```python
from build123d import *

# Parameters (mm, degrees)
ODEBRAT_VYSUNUT_M1_DEPTH = 2.4
ODEBRAT_VYSUNUT_M2_DEPTH = 2.9
SKICA4_W                 = 43.201709197
SKICA4_H                 = 57.022390215
SKICA4_W_2               = 28.704491345
SKICA4_H_2               = 62.531332999
ODEBRAT_VYSUNUT_M3_DEPTH = 320.0000001
M6_Z_VIT1_D              = 5
M6_Z_VIT1_DEPTH          = 22
M6_Z_VIT1_TIP            = 1.502151548
M5_Z_VIT1_D              = 4.2
M5_Z_VIT1_DEPTH          = 20
M5_Z_VIT1_TIP            = 1.2618073
ZKOSEN_1_SIZE            = 1
ZKOSEN_1_SIZE2           = 0.577350269
ZKOSEN_1_PART_2_SIZE     = 1
ZKOSEN_1_PART_2_SIZE2    = 0.577350269


with BuildPart() as part:
    # Skica1 → Rotovat1 (revolve)
    with BuildSketch(Plane.XY, mode=Mode.PRIVATE) as rotovat1_sk:
        Polygon((0, 0), (0, 6), (39, 6), (39, 5.75), (83.5, 5.75), (83.5, 6), (113.5, 6), (113.5, 5.75), (158, 5.75), (158, 6), (174, 6), (174, 10), (184, 10), (184, 9.75), (286.5, 9.75), (286.5, 10), (310, 10), (310, 12.5), (319, 12.5), (319, 10), (329, 10), (329, 9.75), (570, 9.75), (570, 7.5), (630, 7.5), (630, 6), (642, 6), (642, 0), align=None)
    revolve(rotovat1_sk.sketch.rotate(Axis((-5427.299905209, 0, 0), (1, 0, 0)), 180), axis=Axis((-5427.299905209, 0, 0), (1, 0, 0)))  # turned: the seam where the file's is

    # Skica2 → Odebrat vysunutím1 (cut)
    with BuildSketch(Plane(origin=(0, 6, 0), x_dir=(1, 0, 0), z_dir=(0, 1, 0))):
        with BuildLine():
            Line((6, 2), (18, 2))
            ThreePointArc((18, 2), (20, 0), (18, -2))
            Line((18, -2), (6, -2))
            ThreePointArc((6, -2), (4, 0), (6, 2))
        make_face()
    extrude(amount=-ODEBRAT_VYSUNUT_M1_DEPTH, mode=Mode.SUBTRACT)

    # Skica3 → Odebrat vysunutím2 (cut)
    with BuildSketch(Plane(origin=(0, 7.5, 0), x_dir=(1, 0, 0), z_dir=(0, 1, 0))):
        with BuildLine():
            Line((616, 2.5), (623, 2.5))
            ThreePointArc((623, 2.5), (625.5, 0), (623, -2.5))
            Line((623, -2.5), (616, -2.5))
            ThreePointArc((616, -2.5), (613.5, 0), (616, 2.5))
        make_face()
    extrude(amount=-ODEBRAT_VYSUNUT_M2_DEPTH, mode=Mode.SUBTRACT)

    # Skica4 → Odebrat vysunutím3 (cut, through all)
    with BuildSketch(Plane(origin=(319, 0, 0), x_dir=(0, 0, -1), z_dir=(1, 0, 0))):
        with Locations((-32.600854599, -5.674005363)):
            Rectangle(SKICA4_W, SKICA4_H)
        with Locations((25.352245673, -4.175959518)):
            Rectangle(SKICA4_W_2, SKICA4_H_2)
    extrude(amount=-ODEBRAT_VYSUNUT_M3_DEPTH, mode=Mode.SUBTRACT)

    # M6 závit1
    with Locations(Plane(origin=(642, 0, 0), x_dir=(0, 0, -1), z_dir=(1, 0, 0))):
        with Locations((0, 0)):
            Hole(M6_Z_VIT1_D / 2, depth=M6_Z_VIT1_DEPTH)
            with Locations((0, 0, -(M6_Z_VIT1_DEPTH + M6_Z_VIT1_TIP / 2))):  # 118° drill point
                Cone(0, M6_Z_VIT1_D / 2, M6_Z_VIT1_TIP, mode=Mode.SUBTRACT)

    # M5 závit1
    with Locations(Plane.ZY):
        with Locations((0, 0)):
            Hole(M5_Z_VIT1_D / 2, depth=M5_Z_VIT1_DEPTH)
            with Locations((0, 0, -(M5_Z_VIT1_DEPTH + M5_Z_VIT1_TIP / 2))):  # 118° drill point
                Cone(0, M5_Z_VIT1_D / 2, M5_Z_VIT1_TIP, mode=Mode.SUBTRACT)

    # Zkosení1
    zkosen_1_edges = [part.edges().sort_by_distance(p)[0] for p in [
        (570, 9.75, 0),
    ]]
    zkosen_1_side = [part.faces().sort_by_distance(p)[0] for p in [
        (449.5, 9.75, 0),
    ]]
    chamfer(zkosen_1_edges, length=ZKOSEN_1_SIZE, length2=ZKOSEN_1_SIZE2, reference=zkosen_1_side[0])

    # Zkosení1 part 2
    zkosen_1_part_2_edges = [part.edges().sort_by_distance(p)[0] for p in [
        (174, 10, 0),
    ]]
    zkosen_1_part_2_side = [part.faces().sort_by_distance(p)[0] for p in [
        (179, 10, 0),
    ]]
    chamfer(zkosen_1_part_2_edges, length=ZKOSEN_1_PART_2_SIZE, length2=ZKOSEN_1_PART_2_SIZE2, reference=zkosen_1_part_2_side[0])


solid = part.part
```
Model file for the job. Use its own axes, mm. A direction names the side the tool comes from. Coordinates: 2 decimals unless noted, no trailing zeros. Loops run counter-clockwise (first coordinate to the right, second up) from the corner with the lowest first, then second, coordinate; pieces in that order, holes last. Notation, with made-up numbers: (25, 31) - (75, 31) arc R33 cw to (75, 59) - close; hole circle Ø2 at (0, 13). An arc over 180 degrees is marked (long way). Write item = value, one per line. Start each with the question number.
Item 1: Saw through at A-A, the plane x = 337. List the corners of the cut face in (y, z), then the cut area to 3 significant figures.
Item 2: 3-axis set-ups, long thin cutter, end or side, ignore diameter. For faces 1 (the face through (298, 10, 0)), 2 (the face through (570, 8, 0)), 3 (the face through (0, 3, 0)): which of +Z, -Z, +X, -X, +Y, -Y reach the whole face in a straight line?
Item 3: Drop flat-ended pins along their axis: pin 1 Ø1 at (x, y) = (424, -1.5) entering from -Z; pin 2 Ø8 at (x, z) = (298.5, -4.5) entering from +Y; pin 3 Ø1.5 at (x, z) = (360, -3.5) entering from +Y. Give the stop position or say it passes through.
Item 4: Wall check: probe 1 along X at (y, z) = (1.25, 5.75); probe 2 along Z at (x, y) = (632.25, 0); probe 3 along Z at (x, y) = (11.75, 0). Give the ranges that are in metal, low to high. Write a range as [from, to].
Answers:
q1.outline = circle Ø19.5 at (0, 0)
q1.area = 299 mm2
q2.face_1 = -X
q2.face_2 = +X
q2.face_3 = +Z, -Z, -X, +Y, -Y
q3.pin_1 = -9.7
q3.pin_2 = 9.99
q3.pin_3 = 9.35
q4.probe_1 = [0, 39], [83.5, 113.5], [158, 642]
q4.probe_2 = [-6, -2.5], [2.5, 6]
q4.probe_3 = [-6, -2.1], [2.1, 6]
